from build123d import *

# Parameters (mm, degrees)
F1_DEPTH = 6.096
F3_SIZE  = 2.54


# Not quite as in the source:
# - a feature of the source that left no trace in its solid (it failed there, or was rolled back) is left out


with BuildPart() as f1:
    # F0 (on Front) → F1 (new body)
    with BuildSketch(Plane.XZ):
        Polygon((0, 0), (0, 64.7907108068), (-18.6979882419, 56.9636411965), (-18.6979882419, 0), align=None)
        Polygon((0, -48.266902566), (0, 0), (-18.6979882419, 0), (-30.0037488341, -21.3070102036), (-10.8709232882, -21.3070102036), (-10.8709232882, -48.266902566), align=None)
    extrude(amount=F1_DEPTH)

    # F3
    f3_edges = [f1.edges().sort_by_distance(p)[0] for p in [
        (-18.697988, -6.096, 28.481821),
        (-24.350869, -6.096, -10.653505),
        (-9.348994, -6.096, 60.877176),
        (-9.348994, 0, 60.877176),
        (-18.697988, 0, 28.481821),
        (-24.350869, 0, -10.653505),
    ]]
    chamfer(f3_edges, length=F3_SIZE)


solid = f1.part
Can you work these out from the model? Positions are in its coordinate system, mm. A direction names the side the tool comes from. Round coordinates to 2 decimals unless told otherwise and drop trailing zeros. Order: outer loops, then holes, each group sorted by start corner. A loop starts at its lowest first (then second) coordinate and runs counter-clockwise, first axis right, second up. Notation, with made-up numbers: (-7, 80.25) - (32, 80.25) arc R13 cw to (32, 84.25) - close; hole circle Ø4 at (64.5, 67.5). An arc over 180 degrees is marked (long way). Answer in a Markdown table with one row per item.
(1) For P1, Ø1.1, axis at y = -3, z = 33, coming from the -X side; P2, Ø3, axis at y = -4.5, z = -40.5, coming from the -X side, each with a flat end and sliding along its axis, tell me the tip position at first contact or that it passes through.
From the geometry:
| item | result |
|---|---|
| P1 | stops at x = -18.7 |
| P2 | stops at x = -10.87 |
(2) Suppose I cut it at B-B, the plane x = -4. Please give me the cut outline in (y, z), plus the area to 3 significant figures.
From the geometry:
| item | result |
|---|---|
| outline | (-6.1, -48.27) - (0, -48.27) - (0, 60.36) - (-2.54, 63.12) - (-3.56, 63.12) - (-6.1, 60.36) - close |
| area | 672 mm2 |
(3) Suppose I cut it at C-C, the plane z = 27.5. Please give me the cut outline in (x, y).
From the geometry:
| item | result |
|---|---|
| outline | (-18.7, -3.56) - (-16.16, -6.1) - (0, -6.1) - (0, 0) - (-16.16, 0) - (-18.7, -2.54) - close |
(4) Suppose I cut it at A-A, the plane y = -1.25. Please give me the cut outline in (x, z).
From the geometry:
| item | result |
|---|---|
| outline | (-28.54, -21.31) - (-10.87, -21.31) - (-10.87, -48.27) - (0, -48.27) - (0, 63.39) - (-17.41, 56.11) - (-17.41, -0.32) - close |
(5) Please list where these lines run through material, in increasing order: L1, parallel to X at y = -0.25, z = 11; L2, parallel to Z at x = -3, y = -3; L3, parallel to X at y = -4, z = 16.5. Write a range as from..to.
From the geometry:
| item | result |
|---|---|
| L1 | x = -16.41..0 |
| L2 | z = -48.27..63.53 |
| L3 | x = -18.25..0 |
(6) Suppose I cut it at D-D, the plane z = -23. Please give me the cut outline in (x, y).
From the geometry:
| item | result |
|---|---|
| outline | (-10.87, -6.1) - (0, -6.1) - (0, 0) - (-10.87, 0) - close |
(7) Which directions (+Z, -Z, +X, -X, +Y, -Y) give clear straight access to the entire face, cutting with the end or side of a thin tool? Please do faces 1 (the face through (-17.41, -4.844, 28.569)), 2 (the face through (-17.41, -1.25, 28.57)), 3 (the face through (-21, -3, -21.307)).
From the geometry:
| item | result |
|---|---|
| face 1 | +Z, -X, -Y |
| face 2 | +Z, -X, +Y |
| face 3 | -Z, -X, +Y, -Y |
